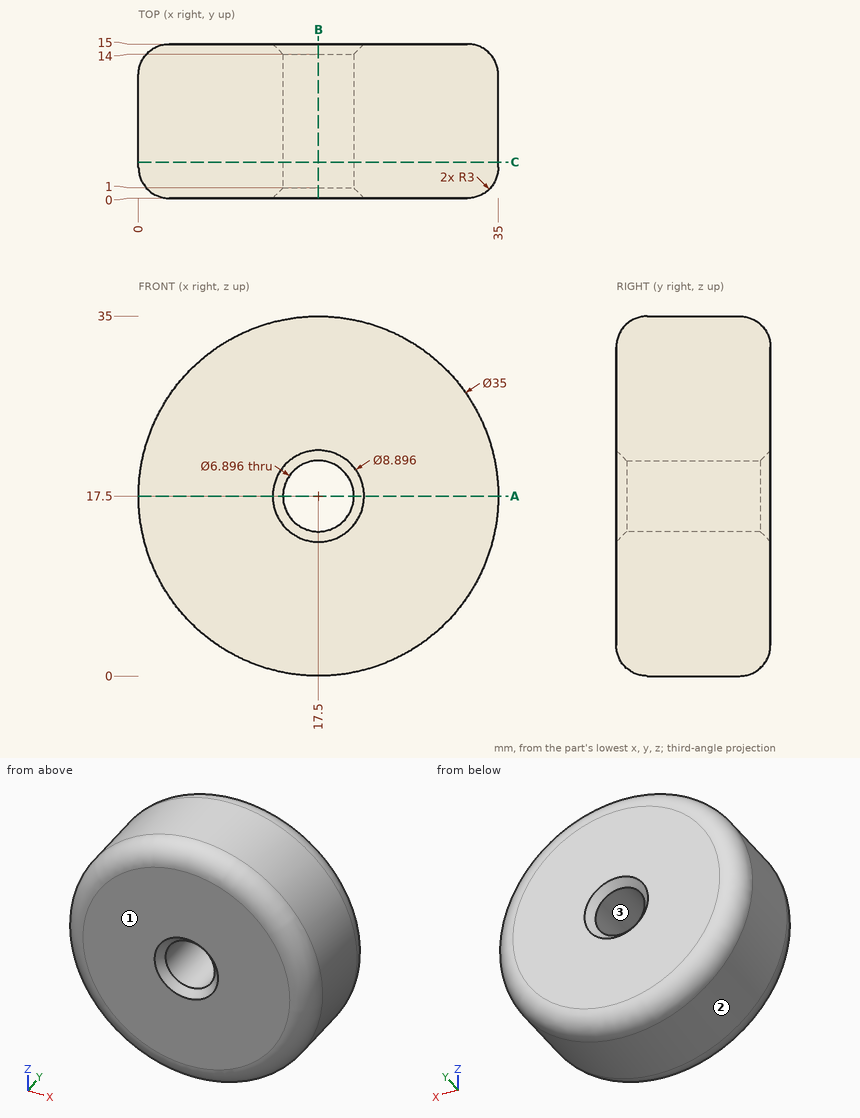
Source: three-view drawing plus pictorial views. Frame: mm from the lowest corner of the part. Give positions to 0.01 mm unless a question says otherwise; leave off trailing zeros. Order: outer loops, then holes, each group sorted by start corner. A loop starts at its lowest first (then second) coordinate and runs counter-clockwise, first axis right, second up. Notation, with made-up numbers: M 59.25,-38 L 95.25,-38 A22 cw 95.25,-18 Z; hole C -39,70 d8. An arc over 180 degrees is marked long. One line per question, with ' | ' between items.
1) Draft query along Z for the marked faces 1, 2 and 3. Return one class per face: pulls with the +Z half, pulls with the -Z half, needs draft (parallel to the pull), parting line crosses it, or undercut.
Filled in:
face 1: needs draft | face 2: parting line crosses it | face 3: undercut
2) Contact query for flat-ended pins moving along their axis: P1, Ø2, axis at x = 27, y = 6.5, coming from the +Z side; P2, Ø1, axis at x = 12.5, y = 8, coming from the +Z side; P3, Ø1, axis at x = 15, y = 3.5, coming from the +Z side. Output: stop coordinate, or through.
Filled in:
P1: stops at z = 32.8 | P2: stops at z = 34.41 | P3: stops at z = 34.89
3) Section A-A on z = 17.5. Output: boundary loops of the cut face in (x, y), and give its area (3 significant figures).
Filled in:
outline: M 0,3 A3 ccw 3,0 L 13.05,0 L 14.05,1 L 14.05,14 L 13.05,15 L 3,15 A3 ccw 0,12 Z; M 20.95,1 L 21.95,0 L 32,0 A3 ccw 35,3 L 35,12 A3 ccw 32,15 L 21.95,15 L 20.95,14 Z | area: 412 mm2
4) Section C-C on y = 3.5. Output: boundary loops of the cut face in (x, z).
Filled in:
outline: C 17.5,17.5 d35; hole C 17.5,17.5 d6.9
5) Section B-B on x = 17.5. Output: boundary loops of the cut face in (y, z), and give its area (3 significant figures).
Filled in:
outline: M 0,3 A3 ccw 3,0 L 12,0 A3 ccw 15,3 L 15,13.05 L 14,14.05 L 1,14.05 L 0,13.05 Z; M 0,21.95 L 1,20.95 L 14,20.95 L 15,21.95 L 15,32 A3 ccw 12,35 L 3,35 A3 ccw 0,32 Z | area: 412 mm2
6) Ray query, L1, parallel to X at y = 5, z = 17.5; L2, parallel to Z at x = 20, y = 7.75; L3, parallel to X at y = 2, z = 17.5. Return the intervals inside material, ascending.
Filled in:
L1: x = 0 to 14.05, 20.95 to 35 | L2: z = 0.18 to 15.13, 19.87 to 34.82 | L3: x = 0.17 to 14.05, 20.95 to 34.83
